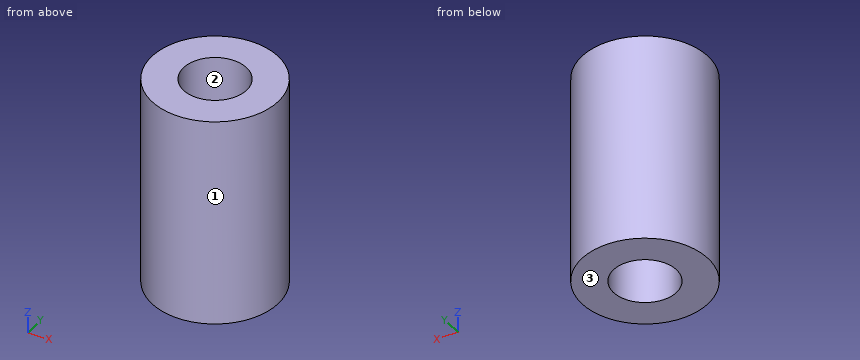
```python
from build123d import *

# Parameters (mm, degrees)
CYLINDER003_R     = 1.5
CYLINDER003_DEPTH = 30
CYLINDER001_R     = 3
CYLINDER001_DEPTH = 10


with BuildPart() as screw_cutout:
    # Cylinder003 → Cylinder003 (new body)
    with BuildSketch(Plane.XY):
        Circle(CYLINDER003_R)
    extrude(amount=CYLINDER003_DEPTH)


with BuildPart() as cut:
    # Cylinder001 → Cylinder001 (new body)
    with BuildSketch(Plane.XY.offset(15)):
        Circle(CYLINDER001_R)
    extrude(amount=CYLINDER001_DEPTH)

    # Cut: cut screw cutout
    add(screw_cutout.part, mode=Mode.SUBTRACT)


solid = cut.part
```
The listing builds one solid part. Answer for the finished solid, in the listing's coordinates (mm). Face numbers are marked on the shaded views. Round coordinates to 2 decimals unless told otherwise and drop trailing zeros. Order: outer loops, then holes, each group sorted by start corner. A loop starts at its lowest first (then second) coordinate and runs counter-clockwise, first axis right, second up. Notation, with made-up numbers: (-19, 26) -> (-2, 26) arc R20 ccw to (-2, 59) -> close; hole circle Ø7 at (-30.5, 45). An arc over 180 degrees is marked (long way). Answer as CSV lines item,"result".
Q1. For a pull along Y with two mould halves and no side action, classify the marked faces 1, 2 and 3 as +Y half, -Y half, draft (parallel to the pull), parting line (faces both ways), or undercut.
Computed values:
face 1,"parting line"
face 2,"undercut"
face 3,"draft"
Q2. Given pin 1 (1 mm diameter, centred on x = -2, z = 22.5, fed in from +Y); pin 2 (2 mm diameter, centred on x = 1.5, z = 18, fed in from -Y); pin 3 (1.5 mm diameter, centred on y = -1.5, z = 20.5, fed in from -X), each flat-ended and moving along its own axis, determine where each tip first touches the part or whether it passes through.
Computed values:
pin 1,"stops at y = 2.6"
pin 2,"stops at y = -2.96"
pin 3,"stops at x = -2.9"
Q3. A cutting plane is placed at A-A on y = 0. Determine the outline of the cut face in (x, z).
Computed values:
outline,"(-3, 15) -> (-1.5, 15) -> (-1.5, 25) -> (-3, 25) -> close; (1.5, 15) -> (3, 15) -> (3, 25) -> (1.5, 25) -> close"
Q4. A cutting plane is placed at C-C on z = 23.75. Determine the outline of the cut face in (x, y).
Computed values:
outline,"circle Ø6 at (0, 0); hole circle Ø3 at (0, 0)"
Q5. Consider line 1 (Y direction, x = 0, z = 18); line 2 (Y direction, x = 1, z = 22.5); line 3 (X direction, y = 1.2, z = 16). Determine where each line is inside the solid, lowest interval first. Write a range as from..to.
Computed values:
line 1,"y = -3..-1.5, 1.5..3"
line 2,"y = -2.83..-1.12, 1.12..2.83"
line 3,"x = -2.75..-0.9, 0.9..2.75"
Q6. A cutting plane is placed at D-D on y = -2.5. Determine the outline of the cut face in (x, z).
Computed values:
outline,"(-1.66, 15) -> (1.66, 15) -> (1.66, 25) -> (-1.66, 25) -> close"
